Can you work these out from the drawing? Everything is in mm from the part's minimum corner. Coordinates: 2 decimals unless noted, no trailing zeros. Loops run counter-clockwise (first coordinate to the right, second up) from the corner with the lowest first, then second, coordinate; pieces in that order, holes last. Notation, with made-up numbers: M 45,57.5 L 60,57.5 A18 cw 60,72.5 Z; hole C -15,23.5 d7. An arc over 180 degrees is marked long. Write each question's results on one line, items separated by ' | '.
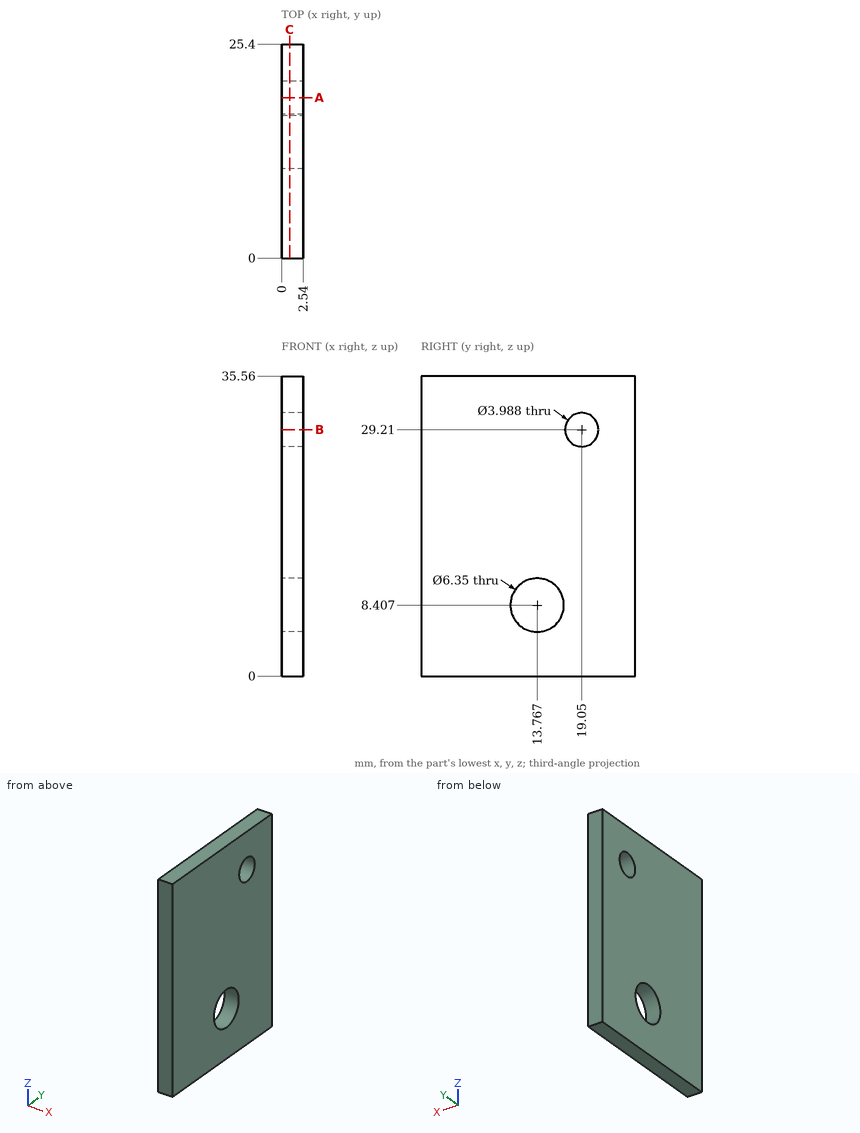
(1) Imagine slicing it at B-B, the plane z = 29.21. List the corners of the cut face in (x, y) for me.
Reported:
outline: M 0,0 L 2.54,0 L 2.54,17.06 L 0,17.06 Z; M 0,21.04 L 2.54,21.04 L 2.54,25.4 L 0,25.4 Z
(2) Please list where these lines run through material, in increasing order: probe 1 along Z at (x, y) = (1.8, 19); probe 2 along Y at (x, z) = (0.15, 5.5) (1 decimal); probe 3 along Y at (x, z) = (1.4, 29). Write a range as from..to.
Reported:
probe 1: z = 0..27.22, 31.2..35.56 | probe 2: y = 0..12.5, 15..25.4 | probe 3: y = 0..17.07, 21.03..25.4
(3) Imagine slicing it at A-A, the plane y = 19.05. List the corners of the cut face in (x, z) for me.
Reported:
outline: M 0,0 L 2.54,0 L 2.54,27.22 L 0,27.22 Z; M 0,31.2 L 2.54,31.2 L 2.54,35.56 L 0,35.56 Z
(4) Imagine slicing it at C-C, the plane x = 0.95. State how many separate pieces and enclosed holes the cut face has, and give its area (3 significant figures).
Reported:
separate pieces: 1 | enclosed holes: 2 | area: 859 mm2
